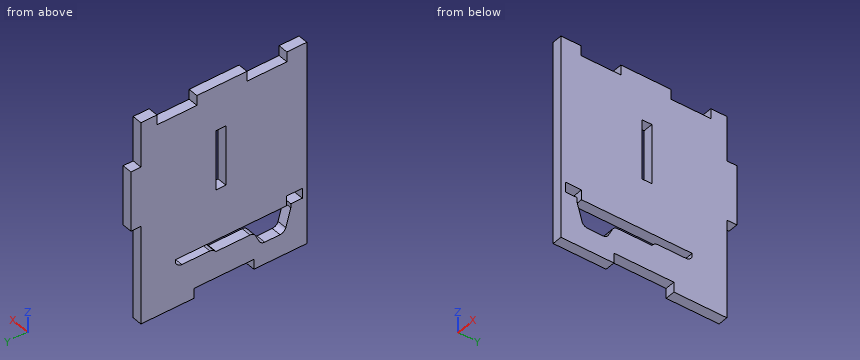
```python
from build123d import *

# Parameters (mm, degrees)
SKETCH_1_W      = 30
SKETCH_1_H      = 5
EXTRUDE_1_DEPTH = 5


with BuildPart() as part:
    # 草图1 → 凸台-拉伸1 (new body)
    with BuildSketch(Plane(origin=(0, 0, 0), x_dir=(0, 0, -1), z_dir=(1, 0, 0))):
        Polygon((-71.794387691, -30.467986568), (30.205612309, -30.467986568), (30.205612309, -3.967986568), (25.205612309, -3.967986568), (25.205612309, 26.032013432), (30.205612309, 26.032013432), (30.205612309, 52.532013432), (-19.294387691, 52.532013432), (-19.294387691, 57.532013432), (-49.294387691, 57.532013432), (-49.294387691, 52.532013432), (-71.794387691, 52.532013432), (-71.794387691, 44.532013432), (-66.794387691, 44.532013432), (-66.794387691, 24.532013432), (-71.794387691, 24.532013432), (-71.794387691, -0.467986568), (-66.794387691, -0.467986568), (-66.794387691, -20.467986568), (-71.794387691, -20.467986568), align=None)
        with Locations((-34.294387691, 12.532013432)):
            Rectangle(SKETCH_1_W, SKETCH_1_H, mode=Mode.SUBTRACT)
        with BuildLine():
            Line((6.101172562, -20.197681499), (6.101172562, 35.190002139))
            Line((6.101172562, 35.190002139), (8.101172562, 35.190013424))
            Line((8.101172562, 35.190013424), (9.065260801, 34.381164181))
            ThreePointArc((9.065260801, 34.381164181), (9.8559397, 33.350845179), (10.137061428, 32.082893705))
            Line((10.137061428, 32.082893705), (10.137061428, 18.013655336))
            ThreePointArc((10.137061428, 18.013655336), (10.36542283, 16.865605039), (11.015741084, 15.892334992))
            Line((11.015741084, 15.892334992), (11.926129512, 14.981946565))
            Line((11.926129512, 14.981946565), (11.926129512, -2.055830909))
            ThreePointArc((11.926129512, -2.055830909), (12.372134093, -3.629713816), (13.577534447, -4.735624064))
            Line((13.577534447, -4.735624064), (17.504207374, -6.71170633))
            ThreePointArc((17.504207374, -6.71170633), (18.709607728, -7.817616578), (19.155612309, -9.391499485))
            Line((19.155612309, -9.391499485), (19.155612309, -17.062905379))
            ThreePointArc((19.155612309, -17.062905379), (18.550098161, -18.870234212), (16.977987304, -19.947987591))
            Line((16.977987304, -19.947987591), (8.137246436, -22.467986568))
            Line((8.137246436, -22.467986568), (6.137246436, -22.467986568))
            Line((6.137246436, -22.467986568), (6.137246436, -28.197986568))
            Line((6.137246436, -28.197986568), (1.137246436, -28.197986568))
            Line((1.137246436, -28.197986568), (1.137246436, -20.197681499))
            Line((1.137246436, -20.197681499), (6.101172562, -20.197681499))
        make_face(mode=Mode.SUBTRACT)
    extrude(amount=EXTRUDE_1_DEPTH)


solid = part.part
```
Geometry: final body of the model. Coordinates: model frame, mm. Coordinates: 2 decimals unless noted, no trailing zeros. Loops run counter-clockwise (first coordinate to the right, second up) from the corner with the lowest first, then second, coordinate; pieces in that order, holes last. Notation, with made-up numbers: (-1.75, 74) -> (24.25, 74) arc R32 cw to (24.25, 101) -> close; hole circle Ø8 at (-1.5, 39.25). An arc over 180 degrees is marked (long way). Use a Markdown table: item, result. Add a question column.
(1) Section query C-C, the plane x = 1.05. State how many separate pieces and enclosed holes the cut face has, plus the area to 3 significant figures.
(2) Pin query (flat end, axial travel): pin 1 Ø5 at (y, z) = (33, -7.5) entering from -X; pin 2 Ø1.5 at (x, z) = (1.5, -28.5) entering from +Y. Return the tip coordinate at first contact, or that it passes through.
(3) Section query D-D, the plane z = -22.5. Return loops of the section in (x, y), plus the area to 3 significant figures.
(4) Line query: line 1 along Y through (x, z) = (2.7, 38); line 2 along Z through (x, y) = (3.85, 5.5); line 3 along Z through (x, y) = (1.65, -14.5). Output: solid intervals per line, ascending.
(5) Section query A-A, the plane z = 48. Return loops of the section in (x, y), plus the area to 3 significant figures.
(6) Section query B-B, the plane y = 4.5. Return loops of the section in (x, z), plus the area to 3 significant figures.
Answer:
| question | item | result |
|---|---|---|
| 1 | separate pieces | 1 |
| 1 | enclosed holes | 2 |
| 1 | area | 7,670 mm^2 |
| 2 | pin 1 | stops at x = 0 |
| 2 | pin 2 | stops at y = 52.53 |
| 3 | outline | (0, -30.47) -> (5, -30.47) -> (5, 52.53) -> (0, 52.53) -> close |
| 3 | area | 415 mm^2 |
| 4 | line 1 | y = -30.47 to 10.03, 15.03 to 57.53 |
| 4 | line 2 | z = -25.21 to -11.93, -6.1 to 71.79 |
| 4 | line 3 | z = -30.21 to -19.16, -6.1 to 66.79 |
| 5 | outline | (0, -30.47) -> (5, -30.47) -> (5, 10.03) -> (0, 10.03) -> close; (0, 15.03) -> (5, 15.03) -> (5, 57.53) -> (0, 57.53) -> close |
| 5 | area | 415 mm^2 |
| 6 | outline | (0, -25.21) -> (5, -25.21) -> (5, -11.93) -> (0, -11.93) -> close; (0, -6.1) -> (5, -6.1) -> (5, 71.79) -> (0, 71.79) -> close |
| 6 | area | 456 mm^2 |
